Read the model definition and answer for the solid it produces. Units are mm, in the model's axes. A direction names the side the tool comes from. Round coordinates to 2 decimals unless told otherwise and drop trailing zeros. Write each loop counter-clockwise with the first axis right and the second up, starting at its lowest first coordinate (ties: lowest second). Pieces come first, ordered by that corner, then holes. Notation, with made-up numbers: (54, -28) -> (113, -28) arc R25 cw to (113, 9) -> close; hole circle Ø2 at (40, 50.5). An arc over 180 degrees is marked (long way). Return JSON: item names as keys, results as strings. Group by question number.
(1) A cutting plane is placed at C-C on x = 12. Give the vertices of the cut face in (y, z), then the cut area to 3 significant figures.
(2) Straight lines are drawn through the part: line 1 (Z direction, x = 0, y = 2.2); line 2 (X direction, y = 5.95, z = -54.5); line 3 (Z direction, x = -12, y = 6.6). For each, find the intervals that lie inside material, in ascending order.
(3) A cutting plane is placed at B-B on y = 5.75. Give the vertices of the cut face in (x, z).
(4) For faces 1 (the flat face through (14, 3.5, -53)), 2 (the cylindrical face through (1.63, 2.17, -62.18)), 3 (the flat face through (18, 4, 1)), determine the directions among +Z, -Z, +X, -X, +Y, -Y from which every point of the face is accessible in a straight line to the end or side of a thin tool.
(5) The mould has two halves that part along Z. Classify faces 4 (the flat face through (0, 0, -1)), 5 (the cylindrical face through (-15.2, 5.5, -2.1)), 6 (the flat face through (0, 4, 99.5)): released by +Z, released by -Z, zero draft, split by the parting line, or undercut.
(6) Given pin 1 (4 mm diameter, centred on x = -14, z = -3.5, fed in from +Y); pin 2 (6 mm diameter, centred on x = -12, z = -4.5, fed in from +Y), each flat-ended and moving along its own axis, determine where each tip first touches the part or whether it passes through.
(7) A cutting plane is placed at A-A on z = -4.5. Give the vertices of the cut face in (x, y).
(8) A cutting plane is placed at D-D on x = 0. State how many separate pieces and enclosed holes the cut face has, then the cut area to 3 significant figures.
```python
from build123d import *

# Parameters (mm, degrees)
SKETCH1_W                       = 36
SKETCH1_H                       = 199
BOSS_EXTRUDE1_DEPTH             = 7.5
CBORE_FOR_M4_SHCS1_D            = 4.5
CBORE_FOR_M4_SHCS1_CBORE_D      = 8
CBORE_FOR_M4_SHCS1_CBORE_DEPTH  = 4
CHAMFER1_SIZE                   = 1
CBORE_FOR_M8_SBHCS1_D           = 9
CBORE_FOR_M8_SBHCS1_CBORE_D     = 15
CBORE_FOR_M8_SBHCS1_CBORE_DEPTH = 4.4


with BuildPart() as part:
    # Sketch1 → Boss-Extrude1 (new body)
    with BuildSketch(Plane(origin=(0, 0, 0), x_dir=(1, 0, 0), z_dir=(0, 1, 0))):
        Rectangle(SKETCH1_W, SKETCH1_H)
    extrude(amount=BOSS_EXTRUDE1_DEPTH)

    # CBORE for M4 SHCS1 (through all)
    with Locations(Plane(origin=(0, 7.5, 0), x_dir=(1, 0, 0), z_dir=(0, 1, 0))):
        with Locations((-12, 54.5), (12, 54.5), (12, 4.5), (-12, 4.5)):
            CounterBoreHole(CBORE_FOR_M4_SHCS1_D / 2, CBORE_FOR_M4_SHCS1_CBORE_D / 2, CBORE_FOR_M4_SHCS1_CBORE_DEPTH)

    # Chamfer1
    chamfer1_edges = [part.edges().sort_by_distance(p)[0] for p in [
        (0, 0, 99.5),
        (-18, 0, 0),
        (0, 0, -99.5),
        (18, 0, 0),
        (18, 3.75, 99.5),
        (-18, 3.75, 99.5),
        (-18, 3.75, -99.5),
        (18, 3.75, -99.5),
    ]]
    chamfer(chamfer1_edges, length=CHAMFER1_SIZE)

    # CBORE for M8 SBHCS1 (through all)
    with Locations(Plane(origin=(0, 0, 0), x_dir=(-1, 0, 0), z_dir=(0, -1, 0))):
        with Locations((0, 69.5), (0, -10.5), (0, -70.5)):
            CounterBoreHole(CBORE_FOR_M8_SBHCS1_D / 2, CBORE_FOR_M8_SBHCS1_CBORE_D / 2, CBORE_FOR_M8_SBHCS1_CBORE_DEPTH)


solid = part.part
```
Checks:
{
 "1": {"outline": "(0, -98.5) -> (1, -99.5) -> (7.5, -99.5) -> (7.5, -58.5) -> (3.5, -58.5) -> (3.5, -56.75) -> (0, -56.75) -> close; (0, -52.25) -> (3.5, -52.25) -> (3.5, -50.5) -> (7.5, -50.5) -> (7.5, -8.5) -> (3.5, -8.5) -> (3.5, -6.75) -> (0, -6.75) -> close; (0, -2.25) -> (3.5, -2.25) -> (3.5, -0.5) -> (7.5, -0.5) -> (7.5, 99.5) -> (1, 99.5) -> (0, 98.5) -> close", "area": "1,400 mm^2"},
 "2": {"line 1": "z = -99.5 to -77, -62 to 3, 18 to 63, 78 to 99.5", "line 2": "x = -18 to -16, -8 to 8, 16 to 18", "line 3": "z = -99.5 to -58.5, -50.5 to -8.5, -0.5 to 99.5"},
 "3": {"outline": "(-18, -98.5) -> (-17, -99.5) -> (17, -99.5) -> (18, -98.5) -> (18, 98.5) -> (17, 99.5) -> (-17, 99.5) -> (-18, 98.5) -> close; hole circle Ø8 at (-12, -54.5); hole circle Ø8 at (-12, -4.5); hole circle Ø9 at (0, -69.5); hole circle Ø9 at (0, 10.5); hole circle Ø9 at (0, 70.5); hole circle Ø8 at (12, -54.5); hole circle Ø8 at (12, -4.5)"},
 "4": {"face 1": "+Y", "face 2": "-Y", "face 3": "+Z, -Z, +X, +Y, -Y"},
 "5": {"face 4": "zero draft", "face 5": "undercut", "face 6": "released by +Z"},
 "6": {"pin 1": "stops at y = 7.5", "pin 2": "stops at y = 3.5"},
 "7": {"outline": "(-18, 1) -> (-17, 0) -> (-14.25, 0) -> (-14.25, 3.5) -> (-16, 3.5) -> (-16, 7.5) -> (-18, 7.5) -> close; (-9.75, 0) -> (9.75, 0) -> (9.75, 3.5) -> (8, 3.5) -> (8, 7.5) -> (-8, 7.5) -> (-8, 3.5) -> (-9.75, 3.5) -> close; (14.25, 0) -> (17, 0) -> (18, 1) -> (18, 7.5) -> (16, 7.5) -> (16, 3.5) -> (14.25, 3.5) -> close"},
 "8": {"separate pieces": "4", "enclosed holes": "0", "area": "1,210 mm^2"}
}
